The model under review builds one solid part; all positions refer to its coordinate system, in mm. Round coordinates to 2 decimals unless told otherwise and drop trailing zeros. Write each loop counter-clockwise with the first axis right and the second up, starting at its lowest first coordinate (ties: lowest second). Pieces come first, ordered by that corner, then holes.
Item 1: To check wall thickness, follow L1, parallel to Y at x = -5, z = 0.35; L2, parallel to X at y = 2.5, z = 0.35; L3, parallel to Y at x = -12, z = 0.1. State the ranges of each line that lie inside material, in increasing order.
Item 2: Add section A-A (z = 0.35). Give the boundary of the cut face in (x, y).
Item 3: Add section D-D (y = 6.5). Give the boundary of the cut face in (x, z), plus the area to 3 significant figures.
Item 4: Add section C-C (x = 4). Give the boundary of the cut face in (y, z).
Item 5: Add section B-B (y = -3.5). Give the boundary of the cut face in (x, z), plus the area to 3 significant figures.
```python
from build123d import *

# Parameters (mm, degrees)
SKETCH_1_W      = 16
SKETCH_1_H      = 2
EXTRUDE_1_DEPTH = 0.5


with BuildPart() as part:
    # 草图1 → 凸台-拉伸1 (new body)
    with BuildSketch(Plane.XY):
        Polygon((-14, 5.5), (-11, 8.5), (11, 8.5), (14, 5.5), (14, -5.5), (11, -8.5), (-11, -8.5), (-14, -5.5), align=None)
        with Locations((0, 3)):
            Rectangle(SKETCH_1_W, SKETCH_1_H, mode=Mode.SUBTRACT)
        with Locations((0, -3)):
            Rectangle(SKETCH_1_W, SKETCH_1_H, mode=Mode.SUBTRACT)
    extrude(amount=EXTRUDE_1_DEPTH)


solid = part.part
```
Numbers:
1. L1: y = -8.5 to -4, -2 to 2, 4 to 8.5
1. L2: x = -14 to -8, 8 to 14
1. L3: y = -7.5 to 7.5
2. outline: (-14, -5.5) - (-11, -8.5) - (11, -8.5) - (14, -5.5) - (14, 5.5) - (11, 8.5) - (-11, 8.5) - (-14, 5.5) - close; hole (-8, -4) - (8, -4) - (8, -2) - (-8, -2) - close; hole (-8, 2) - (8, 2) - (8, 4) - (-8, 4) - close
3. outline: (-13, 0) - (13, 0) - (13, 0.5) - (-13, 0.5) - close
3. area: 13.0 mm2
4. outline: (-8.5, 0) - (-4, 0) - (-4, 0.5) - (-8.5, 0.5) - close; (-2, 0) - (2, 0) - (2, 0.5) - (-2, 0.5) - close; (4, 0) - (8.5, 0) - (8.5, 0.5) - (4, 0.5) - close
5. outline: (-14, 0) - (-8, 0) - (-8, 0.5) - (-14, 0.5) - close; (8, 0) - (14, 0) - (14, 0.5) - (8, 0.5) - close
5. area: 6.00 mm2
